```python
from build123d import *

# Parameters (mm, degrees)
BOSS_EXTRUDE1_OUTLINE_R = 2.2479
BOSS_EXTRUDE1_DEPTH     = 2
FILLET1_R               = 0.508


# Read off the part's stored shape, not the designer's step: Boss-Extrude1
with BuildPart() as part:
    # Boss-Extrude1 outline → Boss-Extrude1 (new body)
    with BuildSketch(Plane.XY.offset(-4.3)):
        with BuildLine():
            Line((-3.665078359, -78.538329641), (9.376516015, -4.575772565))
            ThreePointArc((9.376516015, -4.575772565), (7.222943475, -8.305869622), (3.175551027, -9.779))
            Line((3.175551027, -9.779), (-71.734942292, -9.779))
            ThreePointArc((-71.734942292, -9.779), (-73.054687902, -9.923572648), (-74.311835376, -10.350433227))
            Line((-74.311835376, -10.350433227), (-151.921287837, -46.550785133))
            ThreePointArc((-151.921287837, -46.550785133), (-156.284298691, -46.904620517), (-159.820994296, -44.325309098))
            ThreePointArc((-159.820994296, -44.325309098), (-158.24873565, -46.442088317), (-156.273248149, -48.188570679))
            Line((-156.273248149, -48.188570679), (-130.476004779, -66.603469659))
            ThreePointArc((-130.476004779, -66.603469659), (-122.742535166, -73.406833136), (-116.540360394, -81.630295604))
            Line((-116.540360394, -81.630295604), (-113.642182841, -86.414778297))
            ThreePointArc((-113.642182841, -86.414778297), (-99.756521843, -99.869092495), (-81.054590835, -104.775))
            Line((-81.054590835, -104.775), (-34.932724517, -104.775))
            ThreePointArc((-34.932724517, -104.775), (-14.52421791, -97.346911069), (-3.665078359, -78.538329641))
        make_face()
        with Locations((-142.126033439, -49.549218379)):
            Circle(BOSS_EXTRUDE1_OUTLINE_R, mode=Mode.SUBTRACT)
        with Locations((0.028082134, -16.637)):
            Circle(BOSS_EXTRUDE1_OUTLINE_R, mode=Mode.SUBTRACT)
    extrude(amount=BOSS_EXTRUDE1_DEPTH)

    # Fillet1
    fillet1_edges = [part.edges().sort_by_distance(p)[0] for p in [
        (9.376516015, -4.575772565, -3.3),
        (-159.820994296, -44.325309098, -3.3),
    ]]
    fillet(fillet1_edges, radius=FILLET1_R)


solid = part.part
```
Input: part model. Units: mm. Frame: model coordinates. Round coordinates to 2 decimals unless told otherwise and drop trailing zeros. Loops run counter-clockwise (first coordinate to the right, second up) from the corner with the lowest first, then second, coordinate; pieces in that order, holes last. Notation, with made-up numbers: (-31, 8) -> (-9, 8) arc R16 cw to (-9, 13) -> close; hole circle Ø11 at (45.5, 75). An arc over 180 degrees is marked (long way). Use one line per item in the form item = value. Start each with the question number.
Item 1: Section query B-B on y = -72. Return the cut outline in (x, z).
Item 2: Section query C-C on x = -39. Return the cut outline in (y, z) (3 decimals).
Item 3: Section query D-D on z = -2.9. Count the separate pieces of the cut face and the enclosed holes in it, then the cut area to 3 significant figures.
Item 4: Material intervals for L1, parallel to X at y = -16, z = -3.4; L2, parallel to Y at x = -51.5, z = -3.15 (3 decimals); L3, parallel to X at y = -47.5, z = -3.4, sorted ascending. Write a range as from..to.
Item 5: Mould query, pull axis Y, two halves, no side actions, for faces 1 (the face through (-57, -55, -2.3)), 2 (the face through (-140.05, -50.41, -3.31)), 3 (the face through (-122.84, -73.3, -3.31)). Classes: pulls with the +Y half, pulls with the -Y half, needs draft (parallel to the pull), parting line crosses it, or undercut.
Item 6: Contact query for flat-ended pins moving along their axis: pin 1 Ø6 at (x, y) = (-142.13, -49.55) entering from -Z; pin 2 Ø0.6 at (x, z) = (-22, -3.5) entering from +Y. Output: stop coordinate, or through.
Item 7: Section query A-A on x = -142. Return the cut outline in (y, z).
Ans:
q1.outline = (-124.1, -4.3) -> (-2.51, -4.3) -> (-2.51, -2.3) -> (-124.1, -2.3) -> close
q2.outline = (-104.775, -4.3) -> (-9.779, -4.3) -> (-9.779, -2.3) -> (-104.775, -2.3) -> close
q3.separate_pieces = 1
q3.enclosed_holes = 2
q3.area = 11,200 mm^2
q4.L1 = -86.42..-2.13, 2.18..7.36
q4.L2 = -104.775..-9.779
q4.L3 = -157.01..-143.05, -141.2..1.81
q5.face_1 = needs draft
q5.face_2 = undercut
q5.face_3 = pulls with the -Y half
q6.pin_1 = -4.3
q6.pin_2 = -9.78
q7.outline = (-58.38, -4.3) -> (-51.79, -4.3) -> (-51.79, -2.3) -> (-58.38, -2.3) -> close; (-47.3, -4.3) -> (-41.92, -4.3) -> (-41.92, -2.3) -> (-47.3, -2.3) -> close
